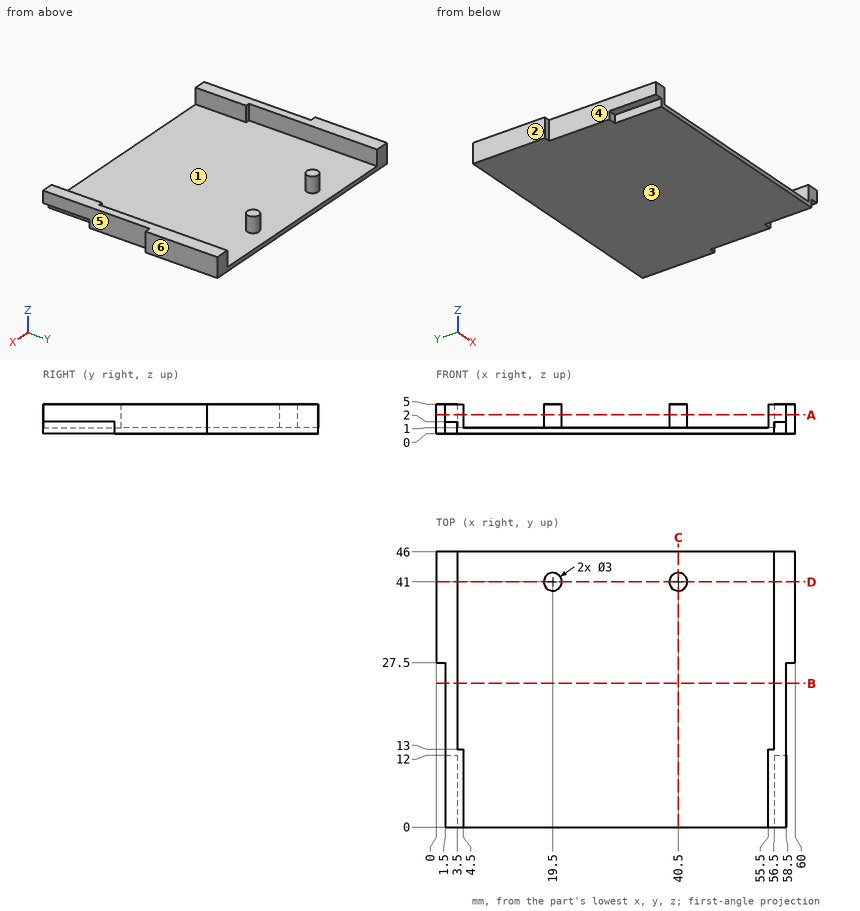
Answer from the drawing. Dimensions are ordinates in mm from the lowest x, y and z of the part. A direction names the side the tool comes from. Round coordinates to 2 decimals unless told otherwise and drop trailing zeros. Write each loop counter-clockwise with the first axis right and the second up, starting at its lowest first coordinate (ties: lowest second). Pieces come first, ordered by that corner, then holes. Notation, with made-up numbers: (-38, -3) -> (1, -3) arc R22 ccw to (1, 35) -> close; hole circle Ø7 at (-25, 55.5). An arc over 180 degrees is marked (long way). Answer in a Markdown table with one row per item. Add a question column.
1) Consider line 1 (X direction, y = 20.5, z = 1.85); line 2 (X direction, y = 10, z = 2.95); line 3 (Z direction, x = 31.5, y = 19.5). Determine where each line is inside the solid, lowest interval first.
2) Determine the mould class of the marked faces 1, 2 and 3 for opening direction X: pulls with the +X half, pulls with the -X half, needs draft (parallel to the pull), parting line crosses it, or undercut.
3) Find section A-A, the plane z = 3.2. Determine the outline of the cut face in (x, y), and give its area (3 significant figures).
4) Find section D-D, the plane y = 41. Determine the outline of the cut face in (x, z), and give its area (3 significant figures).
5) Given P1, Ø2, axis at y = 8.5, z = 1.5, coming from the -X side; P2, Ø10, axis at x = 16.5, y = 19.5, coming from the +Z side; P3, Ø0.8, axis at x = 59.5, z = 2.5, coming from the -Y side; P4, Ø3, axis at x = 9.5, z = 1, coming from the -Y side, each flat-ended and moving along its own axis, determine where each tip first touches the part or whether it passes through.
6) Find section B-B, the plane y = 24. Determine the outline of the cut face in (x, z).
7) Find section C-C, the plane x = 40.5. Determine the outline of the cut face in (y, z), and give its area (3 significant figures).
8) Which of the six approach directions +Z, -Z, +X, -X, +Y, -Y give full straight-line access (tool end or side, diameter ignored) to the marked faces 4, 5 and 6?
Findings below:
| question | item | result |
|---|---|---|
| 1 | line 1 | 1.5 to 3.5, 56.5 to 58.5 |
| 1 | line 2 | 1.5 to 4.5, 55.5 to 58.5 |
| 1 | line 3 | 0 to 1 |
| 2 | face 1 | undercut |
| 2 | face 2 | pulls with the -X half |
| 2 | face 3 | needs draft |
| 3 | outline | (0, 27.5) -> (1.5, 27.5) -> (1.5, 0) -> (4.5, 0) -> (4.5, 13) -> (3.5, 13) -> (3.5, 46) -> (0, 46) -> close; circle Ø3 at (19.5, 41); circle Ø3 at (40.5, 41); (55.5, 0) -> (58.5, 0) -> (58.5, 27.5) -> (60, 27.5) -> (60, 46) -> (56.5, 46) -> (56.5, 13) -> (55.5, 13) -> close |
| 3 | area | 280 mm² |
| 4 | outline | (0, 0) -> (60, 0) -> (60, 5) -> (56.5, 5) -> (56.5, 1) -> (42, 1) -> (42, 5) -> (39, 5) -> (39, 1) -> (21, 1) -> (21, 5) -> (18, 5) -> (18, 1) -> (3.5, 1) -> (3.5, 5) -> (0, 5) -> close |
| 4 | area | 112 mm² |
| 5 | P1 | x = 1.5 |
| 5 | P2 | z = 1 |
| 5 | P3 | y = 27.5 |
| 5 | P4 | y = 0 |
| 6 | outline | (1.5, 0) -> (58.5, 0) -> (58.5, 5) -> (56.5, 5) -> (56.5, 1) -> (3.5, 1) -> (3.5, 5) -> (1.5, 5) -> close |
| 7 | outline | (0, 0) -> (46, 0) -> (46, 1) -> (42.5, 1) -> (42.5, 5) -> (39.5, 5) -> (39.5, 1) -> (0, 1) -> close |
| 7 | area | 58.0 mm² |
| 8 | face 4 | +Z, -Z, -X, -Y |
| 8 | face 5 | +Z, -Z, +X, -Y |
| 8 | face 6 | +Z, -Z, +X, +Y, -Y |
